Autodesk Inventor part; units mm, degrees
ref_plane "YZ Plane" through (0, 0, 0) normal (1, 0, 0) x (0, 1, 0)
ref_plane "XZ Plane" through (0, 0, 0) normal (0, 1, 0) x (-1, 0, 0)
ref_plane "XY Plane" through (0, 0, 0) normal (0, 0, 1) x (1, 0, 0)
sketch "Sketch1" plane through (0, 0, 0) normal (0, 0, 1) x (1, 0, 0)
  line L0 (21.997, 0) -> (10.9985, -19.05)
  line L1 (10.9985, -19.05) -> (-10.9985, -19.05)
  line L2 (-10.9985, -19.05) -> (-21.997, 0)
  line L3 (-21.997, 0) -> (-10.9985, 19.05)
  line L4 (-10.9985, 19.05) -> (10.9985, 19.05)
  line L5 (10.9985, 19.05) -> (21.997, 0)
  circle A0 centre (0, 0) radius 7.9375
  line L6 (8.2489, 14.2875) -> (16.4978, 0) construction
  line L7 (16.4978, 0) -> (8.2489, -14.2875) construction
  line L8 (8.2489, -14.2875) -> (-8.2489, -14.2875) construction
  line L9 (-8.2489, -14.2875) -> (-16.4978, 0) construction
  line L10 (-16.4978, 0) -> (-8.2489, 14.2875) construction
  line L11 (-8.2489, 14.2875) -> (8.2489, 14.2875) construction
  circle A1 centre (-8.2489, 14.2875) radius 2.4384
  circle A2 centre (16.4978, 0) radius 2.4384
  circle A3 centre (-8.2489, -14.2875) radius 2.4384
  dimension "d0" = 15.875
  dimension "d1" = 38.1
  dimension "d2" = 28.575
  dimension "d3" = 4.8768
extrude "Extrusion1" add sketch "Sketch1" along normal blind 25.4
sketch "Sketch2" plane through (0, 0, 25.4) normal (0, 0, 1) x (1, 0, 0)
  circle A0 centre (0, 0) radius 7.9375
  circle A1 centre (0, 0) radius 11.1125
  dimension "d6" = 22.225
extrude "Extrusion2" cut sketch "Sketch2" against normal blind 6.35
sketch "Sketch3" plane through (0, 0, 0) normal (0, 0, -1) x (-1, 0, 0)
  circle A0 centre (0, 0) radius 7.9375
  circle A1 centre (0, 0) radius 11.1125
  dimension "d9" = 22.225
extrude "Extrusion3" cut sketch "Sketch3" against normal blind 6.35
properties part number "BearingBlock" material "Aluminum-6061"
Model file for the job. Use its own axes, mm. A direction names the side the tool comes from. Give positions to 0.01 mm unless a question says otherwise; leave off trailing zeros. Order: outer loops, then holes, each group sorted by start corner. A loop starts at its lowest first (then second) coordinate and runs counter-clockwise, first axis right, second up. Notation, with made-up numbers: (43, -17) - (56, -17) arc R38 ccw to (56, 22) - close; hole circle Ø6 at (43, 43.25). An arc over 180 degrees is marked (long way). Return JSON: item names as keys, results as strings.
1) Cut at B-B, the plane y = -4.5. Give the cut face in (x, z).
Geometry says:
{"outline": "(-19.4, 0) - (-10.16, 0) - (-10.16, 6.35) - (-6.54, 6.35) - (-6.54, 19.05) - (-10.16, 19.05) - (-10.16, 25.4) - (-19.4, 25.4) - close; (6.54, 6.35) - (10.16, 6.35) - (10.16, 0) - (19.4, 0) - (19.4, 25.4) - (10.16, 25.4) - (10.16, 19.05) - (6.54, 19.05) - close"}
2) Cut at A-A, the plane x = 0. Give the cut face in (y, z), plus the area to 3 significant figures.
Geometry says:
{"outline": "(-19.05, 0) - (-11.11, 0) - (-11.11, 6.35) - (-7.94, 6.35) - (-7.94, 19.05) - (-11.11, 19.05) - (-11.11, 25.4) - (-19.05, 25.4) - close; (7.94, 6.35) - (11.11, 6.35) - (11.11, 0) - (19.05, 0) - (19.05, 25.4) - (11.11, 25.4) - (11.11, 19.05) - (7.94, 19.05) - close", "area": "484 mm²"}
3) Pull direction Y, two halves, no side cores. Call faces 1 (the flat face through (9, -8, 0)), 2 (the cylindrical face through (18.824, -0.732, 12.522)), 3 (the flat face through (-16.575, 9.392, 12.522)), 4 (the cylindrical face through (-1.72, 7.75, 12.61)): pulls with the +Y half, pulls with the -Y half, needs draft (parallel to the pull), parting line crosses it, or undercut.
Geometry says:
{"face 1": "needs draft", "face 2": "undercut", "face 3": "pulls with the +Y half", "face 4": "undercut"}
4) Probe line 1 (Y direction, x = 0, z = 4.25); line 2 (Y direction, x = 0, z = 13); line 3 (X direction, y = -1.5, z = 17). List the from-to ranges inside material, lowest first. Write a range as from..to.
Geometry says:
{"line 1": "-19.05..-11.11, 11.11..19.05", "line 2": "-19.05..-7.94, 7.94..19.05", "line 3": "-21.13..-7.79, 7.79..14.58, 18.42..21.13"}
5) 3-axis set-ups, long thin cutter, end or side, ignore diameter. For faces 5 (the flat face through (16.575, -9.392, 12.522)), 6 (the flat face through (8, 3, 6.35)), 7 (the cylindrical face through (10.6, 3.34, 22.27)): which of +Z, -Z, +X, -X, +Y, -Y reach the whole face in a straight line?
Geometry says:
{"face 5": "+Z, -Z, +X, -Y", "face 6": "-Z", "face 7": "+Z"}
6) Cut at C-C, the plane z = 14. Count the separate pieces of the cut face and the enclosed holes in it, plus the area to 3 significant figures.
Geometry says:
{"separate pieces": "1", "enclosed holes": "4", "area": "1,000 mm²"}
7) Flat gauge pins, fed straight in: P1, Ø6, axis at y = -12.5, z = 6, coming from the -X side; P2, Ø8, axis at y = -8.5, z = 9.5, coming from the +X side; P3, Ø14.5, axis at x = 0, y = 0, coming from the +Z side; P4, Ø1, axis at x = 13.5, z = 11, coming from the +Y side. Where does each tip first touch, or does it go through?
Geometry says:
{"P1": "x = -16.51", "P2": "x = 19.4", "P3": "through", "P4": "y = 15.58"}
